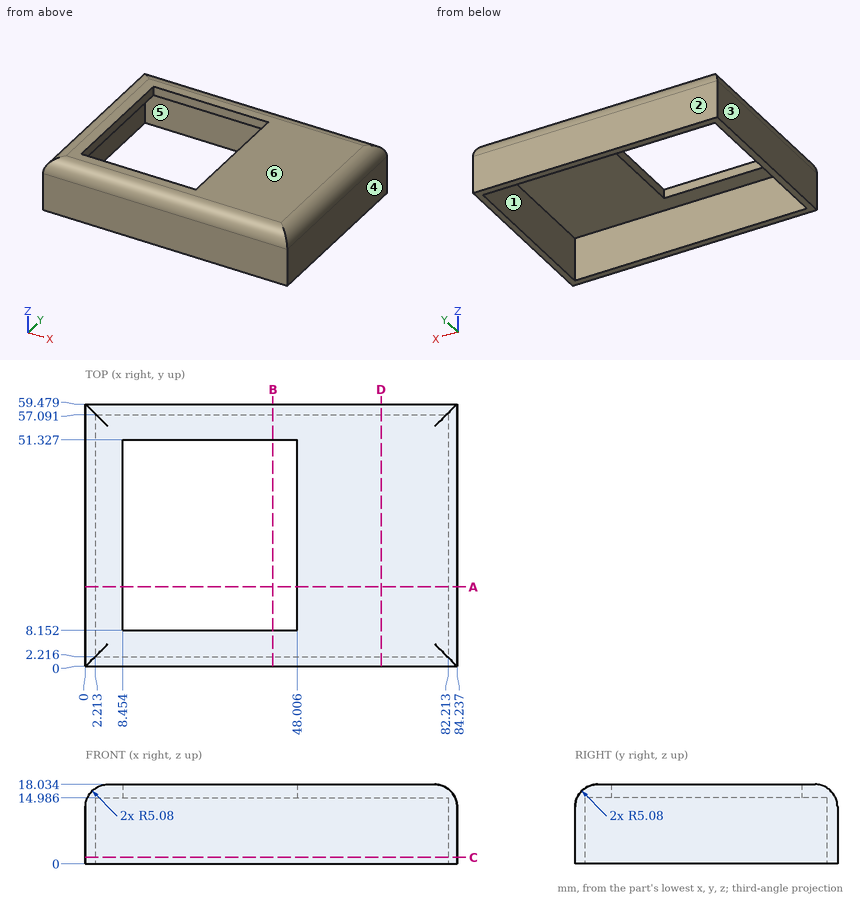
Study the drawing (mm; zero at the part's minimum x, y, z) and answer. A direction names the side the tool comes from. Give positions to 0.01 mm unless a question says otherwise; leave off trailing zeros. Loops run counter-clockwise (first coordinate to the right, second up) from the corner with the lowest first, then second, coordinate; pieces in that order, holes last. Notation, with made-up numbers: (46, -16) -> (65, -16) arc R21 cw to (65, 13) -> close; hole circle Ø4 at (39.25, 74.25). An arc over 180 degrees is marked (long way). Use a Markdown table: item, result. Add a question column.
1) The part is cut by section A-A, the plane y = 18. Determine the outline of the cut face in (x, z).
2) The part is cut by section B-B, the plane x = 42.5. Determine the outline of the cut face in (y, z).
3) The part is cut by section C-C, the plane z = 1.5. Determine the outline of the cut face in (x, y).
4) Each of these flat-tipped pins is pushed along its axis until it touches: P1, Ø2.5, axis at x = 35.5, z = 16.5, coming from the +Y side; P2, Ø2.5, axis at y = 27.5, z = 16, coming from the -X side; P3, Ø3.5, axis at y = 36.5, z = 16.5, coming from the +X side. Where does it stop, or does it pass through?
5) The part is cut by section D-D, the plane x = 67. Determine the outline of the cut face in (y, z).
6) For a pull along X with two mould halves and no side action, classify the marked faces 3, 4, 5 and 6 as +X half, -X half, draft (parallel to the pull), parting line (faces both ways), or undercut.
7) Consider line 1 along Y through (x, z) = (25, 1.5); line 2 along X through (y, z) = (24.5, 12.75); line 3 along Z through (x, y) = (78.5, 9.5). Determine where each line is inside the solid, lowest interval first.
8) Which of the six approach directions +Z, -Z, +X, -X, +Y, -Y give full straight-line access (tool end or side, diameter ignored) to the marked faces 1 and 2?
Reported:
| question | item | result |
|---|---|---|
| 1 | outline | (0, 0) -> (2.21, 0) -> (2.21, 14.99) -> (8.45, 14.99) -> (8.45, 18.03) -> (5.08, 18.03) arc R5.08 ccw to (0, 12.95) -> close; (48.01, 14.99) -> (82.21, 14.99) -> (82.21, 0) -> (84.24, 0) -> (84.24, 12.95) arc R5.08 ccw to (79.16, 18.03) -> (48.01, 18.03) -> close |
| 2 | outline | (0, 0) -> (2.22, 0) -> (2.22, 14.99) -> (8.15, 14.99) -> (8.15, 18.03) -> (5.08, 18.03) arc R5.08 ccw to (0, 12.95) -> close; (51.33, 14.99) -> (57.09, 14.99) -> (57.09, 0) -> (59.48, 0) -> (59.48, 12.95) arc R5.08 ccw to (54.4, 18.03) -> (51.33, 18.03) -> close |
| 3 | outline | (0, 0) -> (84.24, 0) -> (84.24, 59.48) -> (0, 59.48) -> close; hole (2.21, 2.22) -> (82.21, 2.22) -> (82.21, 57.09) -> (2.21, 57.09) -> close |
| 4 | P1 | stops at y = 58.93 |
| 4 | P2 | stops at x = 0.33 |
| 4 | P3 | stops at x = 83.91 |
| 5 | outline | (0, 0) -> (2.22, 0) -> (2.22, 14.99) -> (57.09, 14.99) -> (57.09, 0) -> (59.48, 0) -> (59.48, 12.95) arc R5.08 ccw to (54.4, 18.03) -> (5.08, 18.03) arc R5.08 ccw to (0, 12.95) -> close |
| 6 | face 3 | -X half |
| 6 | face 4 | +X half |
| 6 | face 5 | undercut |
| 6 | face 6 | draft |
| 7 | line 1 | y = 0 to 2.22, 57.09 to 59.48 |
| 7 | line 2 | x = 0 to 2.21, 82.21 to 84.24 |
| 7 | line 3 | z = 14.99 to 18.03 |
| 8 | face 1 | -Z |
| 8 | face 2 | +Z, -Z, +X, -X, +Y |
